Answer from the drawing. Dimensions are ordinates in mm from the lowest x, y and z of the part. A direction names the side the tool comes from. Round coordinates to 2 decimals unless told otherwise and drop trailing zeros. Loops run counter-clockwise (first coordinate to the right, second up) from the corner with the lowest first, then second, coordinate; pieces in that order, holes last. Notation, with made-up numbers: (19, 65.5) - (72, 65.5) arc R22 cw to (72, 75.5) - close; hole circle Ø5 at (-11, 64). An arc over 180 degrees is marked (long way). Answer as CSV lines item,"result".
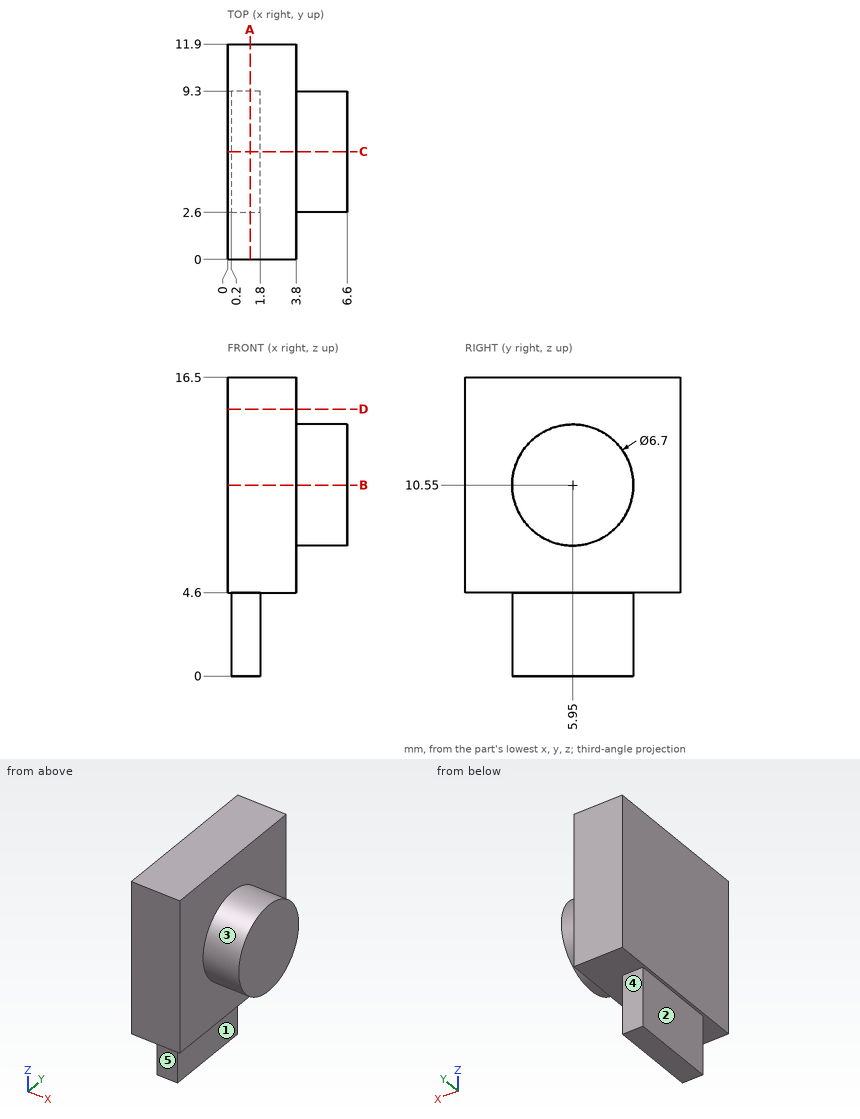
1) A cutting plane is placed at B-B, the plane z = 10.55. Determine the outline of the cut face in (x, y).
Entries:
outline,"(0, 0) - (3.8, 0) - (3.8, 2.6) - (6.6, 2.6) - (6.6, 9.3) - (3.8, 9.3) - (3.8, 11.9) - (0, 11.9) - close"
2) A cutting plane is placed at A-A, the plane x = 1.25. Determine the outline of the cut face in (y, z), plus the area to 3 significant figures.
Entries:
outline,"(0, 4.6) - (2.6, 4.6) - (2.6, 0) - (9.3, 0) - (9.3, 4.6) - (11.9, 4.6) - (11.9, 16.5) - (0, 16.5) - close"
area,"172 mm^2"
3) Each of these flat-tipped pins is pushed along its axis until it touches: P1, Ø2.5, axis at y = 6.5, z = 2, coming from the +X side; P2, Ø1.3, axis at x = 1, z = 1, coming from the +Y side; P3, Ø1.8, axis at x = 1, z = 2.5, coming from the -Y side. Where does it stop, or does it pass through?
Entries:
P1,"stops at x = 1.8"
P2,"stops at y = 9.3"
P3,"stops at y = 2.6"
4) A tool of negligible diameter and unlimited length cuts with its end or side. For the marked faces 1, 2, 3, 4 and 5, from which of +Z, -Z, +X, -X, +Y, -Y can it reach the whole face along a straight path? Write none if from no direction.
Entries:
face 1,"-Z, +X, +Y, -Y"
face 2,"-Z, -X, +Y, -Y"
face 3,"+X"
face 4,"-Z, +X, -X, +Y"
face 5,"-Z, +X, -X, -Y"
5) A cutting plane is placed at C-C, the plane y = 5.95. Determine the outline of the cut face in (x, z).
Entries:
outline,"(0, 4.6) - (0.2, 4.6) - (0.2, 0) - (1.8, 0) - (1.8, 4.6) - (3.8, 4.6) - (3.8, 7.2) - (6.6, 7.2) - (6.6, 13.9) - (3.8, 13.9) - (3.8, 16.5) - (0, 16.5) - close"
6) Find the intervals of material crossed by line 1 (X direction, y = 3, z = 2.5); line 2 (Z direction, x = 2.5, y = 9.25); line 3 (X direction, y = 9.25, z = 6), in increasing order.
Entries:
line 1,"x = 0.2 to 1.8"
line 2,"z = 4.6 to 16.5"
line 3,"x = 0 to 3.8"
7) A cutting plane is placed at D-D, the plane z = 14.75. Determine the outline of the cut face in (x, y).
Entries:
outline,"(0, 0) - (3.8, 0) - (3.8, 11.9) - (0, 11.9) - close"
